```python
from build123d import *

# Parameters (mm, degrees)
SKETCH1_W           = 83.2
SKETCH1_H           = 74.2
BOSS_EXTRUDE1_DEPTH = 15
SHELL1_T            = -2
SKETCH2_W           = 47.9
SKETCH2_H           = 6.5
CUT_EXTRUDE1_DEPTH  = 112.175896668
CUT_EXTRUDE3_DEPTH  = 112.013873007
SKETCH4_W           = 8.2
SKETCH4_H           = 3
CUT_EXTRUDE4_DEPTH  = 112.013873007
SKETCH5_R           = 1.5
CUT_EXTRUDE5_DEPTH  = 113.235823158
SKETCH6_W           = 34.4
SKETCH6_H           = 14.6
CUT_EXTRUDE6_DEPTH  = 113.485021225
BOSS_EXTRUDE2_DEPTH = 12
SKETCH9_W           = 1
SKETCH9_H           = 1.05
EXTRUDE_THIN1_DEPTH = 0.9
FILLET1_R           = 2


with BuildPart() as part:
    # Sketch1 → Boss-Extrude1 (new body)
    with BuildSketch(Plane(origin=(0, 0, 0), x_dir=(1, 0, 0), z_dir=(0, 1, 0))):
        with Locations((41.6, 37.1)):
            Rectangle(SKETCH1_W, SKETCH1_H)
    extrude(amount=BOSS_EXTRUDE1_DEPTH)

    # Shell1
    shell1_openings = [part.faces().sort_by_distance(p)[0] for p in [
        (41.6, 15, -37.1),
    ]]
    offset(amount=SHELL1_T, openings=shell1_openings, kind=Kind.INTERSECTION)

    # Sketch2 → Cut-Extrude1 (cut, through all)
    with BuildSketch(Plane(origin=(0, 0, -2), x_dir=(-1, 0, 0), z_dir=(0, 0, -1))):
        with Locations((-29.95, 11.75)):
            Rectangle(SKETCH2_W, SKETCH2_H)
    extrude(amount=-CUT_EXTRUDE1_DEPTH, mode=Mode.SUBTRACT)

    # Sketch3 → Cut-Extrude3 (cut, through all)
    with BuildSketch(Plane.ZY.offset(-81.2)):
        with BuildLine():
            Line((-13.47, 12.775001119), (-13.47, 13.375))
            Line((-13.47, 13.375), (-13.47, 15))
            Line((-13.47, 15), (-3.73, 15))
            Line((-3.73, 15), (-3.73, 13.375000473))
            Line((-3.73, 13.375000473), (-3.73, 12.774999514))
            ThreePointArc((-3.73, 12.774999514), (-4.222062075, 11.58705914), (-5.410003665, 11.095))
            Line((-5.410003665, 11.095), (-11.79000197, 11.095))
            ThreePointArc((-11.79000197, 11.095), (-12.977940485, 11.5870617), (-13.47, 12.775001119))
        make_face()
    extrude(amount=-CUT_EXTRUDE3_DEPTH, mode=Mode.SUBTRACT)

    # Sketch4 → Cut-Extrude4 (cut, through all)
    with BuildSketch(Plane.ZY.offset(-81.2)):
        with Locations((-18.62, 13.5)):
            Rectangle(SKETCH4_W, SKETCH4_H)
    extrude(amount=-CUT_EXTRUDE4_DEPTH, mode=Mode.SUBTRACT)

    # Sketch5 → Cut-Extrude5 (cut, through all)
    with BuildSketch(Plane(origin=(0, 2, 0), x_dir=(1, 0, 0), z_dir=(0, 1, 0))):
        with Locations(Location((77.9, 27, 0), (0, 0, 270))):
            Circle(SKETCH5_R)
    extrude(amount=-CUT_EXTRUDE5_DEPTH, mode=Mode.SUBTRACT)

    # Sketch6 → Cut-Extrude6 (cut, through all)
    with BuildSketch(Plane.XZ):
        with Locations((26.8, -66.9)):
            Rectangle(SKETCH6_W, SKETCH6_H)
    extrude(amount=-CUT_EXTRUDE6_DEPTH, mode=Mode.SUBTRACT)

    # Sketch7 → Boss-Extrude2 (add)
    with BuildSketch(Plane(origin=(0, 2, 0), x_dir=(1, 0, 0), z_dir=(0, 1, 0))):
        Polygon((44, 72.2), (44, 59.6), (9.6, 59.6), (9.6, 72.2), (8.8, 72.2), (8.8, 58.8), (44.8, 58.8), (44.8, 72.2), align=None)
    extrude(amount=BOSS_EXTRUDE2_DEPTH)

    # Sketch9 → Extrude-Thin1 (add)
    with BuildSketch(Plane(origin=(0, 15, 0), x_dir=(1, 0, 0), z_dir=(0, 1, 0))):
        Polygon((9.6, 72.2), (2, 72.2), (2, 2), (6, 2), (6, 1), (1, 1), (1, 73.2), (9.6, 73.2), align=None)
        Polygon((53.9, 2), (81.2, 2), (81.2, 3.73), (82.2, 3.73), (82.2, 1), (53.9, 1), align=None)
        with Locations((81.7, 13.995)):
            Rectangle(SKETCH9_W, SKETCH9_H)
        Polygon((81.2, 22.72), (81.2, 72.2), (44, 72.2), (44, 73.2), (82.2, 73.2), (82.2, 22.72), align=None)
    extrude(amount=EXTRUDE_THIN1_DEPTH)

    # Fillet1
    fillet1_edges = [part.edges().sort_by_distance(p)[0] for p in [
        (0, 7.5, -74.2),
        (83.2, 7.5, -74.2),
        (83.2, 7.5, 0),
        (0, 7.5, 0),
    ]]
    fillet(fillet1_edges, radius=FILLET1_R)


solid = part.part
```
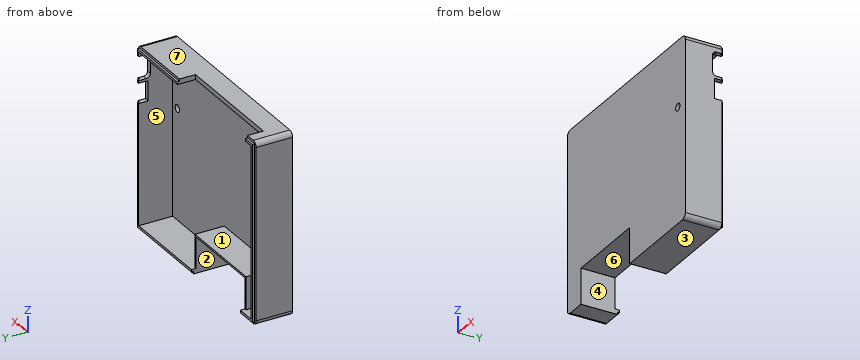
Could you check a few things on this model? Use its own coordinates, in mm. Face numbers are marked on the shaded views. A direction names the side the tool comes from. Round coordinates to 2 decimals unless told otherwise and drop trailing zeros. Write each loop counter-clockwise with the first axis right and the second up, starting at its lowest first coordinate (ties: lowest second). Pieces come first, ordered by that corner, then holes. Notation, with made-up numbers: M 30.5,86 L 69.5,86 A16 cw 69.5,100 Z; hole C 48.5,61.25 d6. An arc over 180 degrees is marked long. Answer in a Markdown table with one row per item. Add a question column.
Q1. Imagine slicing it at B-B (x = 77.9). Please give me the cut outline in (y, z).
Q2. Will these pins go through, and if not, where does the flat tip stop? pin 1 Ø2 at (x, y) = (82.5, 14) entering from -Z; pin 2 Ø3 at (x, z) = (4, -40) entering from +Y; pin 3 Ø1 at (x, z) = (25, -1) entering from +Y; pin 4 Ø0.8 at (x, z) = (82.5, -14) entering from +Y.
Q3. Imagine slicing it at A-A (z = -27). Please give me the cut outline in (x, y).
Q4. Imagine slicing it at C-C (y = 6.5). Please give me the cut outline in (x, z), then the cut area to 3 significant figures.
Q5. Imagine slicing it at D-D (z = -39). Please give me the cut outline in (x, y).
Q6. On a 3-axis mill with a long thin cutter (end or side, diameter ignored), from which of +Z, -Z, +X, -X, +Y, -Y can I reach the whole of each face in a straight line? I mean the marked faces 1, 2 and 3. Say none if no direction works.
Q7. If I drill on line 1 (X direction, y = 5.75, z = -64); line 2 (Z direction, x = 77.9, y = 0.75); line 3 (X direction, y = 1.15, z = -27), over which ranges is the centre line in solid material (lowest first)? Write a range as from..to.
Q8. If we mould it in two halves opening along Z, with no side actions, what happens to the marked faces 4, 5, 6 and 7? For each: +Z half, -Z half, draft (parallel to the pull), parting line (faces both ways), or undercut.
Values:
| question | item | result |
|---|---|---|
| 1 | outline | M 0,-74.2 L 15,-74.2 L 15,-73.2 L 15.9,-73.2 L 15.9,-72.2 L 2,-72.2 L 2,-28.5 L 0,-28.5 Z; M 0,-25.5 L 2,-25.5 L 2,-2 L 15.9,-2 L 15.9,-1 L 15,-1 L 15,0 L 0,0 Z |
| 2 | pin 1 | z = -74.18 |
| 2 | pin 2 | y = 2 |
| 2 | pin 3 | y = 8.5 |
| 2 | pin 4 | y = 15.9 |
| 3 | outline | M 0,0 L 76.4,0 L 76.4,2 L 2,2 L 2,15.9 L 1,15.9 L 1,15 L 0,15 Z; M 79.4,0 L 83.2,0 L 83.2,15 L 82.2,15 L 82.2,15.9 L 81.2,15.9 L 81.2,2 L 79.4,2 Z |
| 4 | outline | M 0,-72.2 A2 ccw 2,-74.2 L 9.6,-74.2 L 9.6,-59.6 L 44,-59.6 L 44,-74.2 L 81.2,-74.2 A2 ccw 83.2,-72.2 L 83.2,-2 A2 ccw 81.2,0 L 2,0 A2 ccw 0,-2 Z; hole M 2,-72.2 L 8.8,-72.2 L 8.8,-58.8 L 44.8,-58.8 L 44.8,-72.2 L 81.2,-72.2 L 81.2,-2 L 2,-2 Z |
| 4 | area | 590 mm^2 |
| 5 | outline | M 0,0 L 83.2,0 L 83.2,15 L 82.2,15 L 82.2,15.9 L 81.2,15.9 L 81.2,2 L 2,2 L 2,15.9 L 1,15.9 L 1,15 L 0,15 Z |
| 6 | face 1 | +Y |
| 6 | face 2 | -Z, +Y, -Y |
| 6 | face 3 | -Z, +X, -X, +Y, -Y |
| 7 | line 1 | 0..2, 8.8..9.6, 44..44.8, 81.2..83.2 |
| 7 | line 2 | -74.2..-28.5, -25.5..0 |
| 7 | line 3 | 0..76.4, 79.4..83.2 |
| 8 | face 4 | draft |
| 8 | face 5 | undercut |
| 8 | face 6 | -Z half |
| 8 | face 7 | +Z half |
